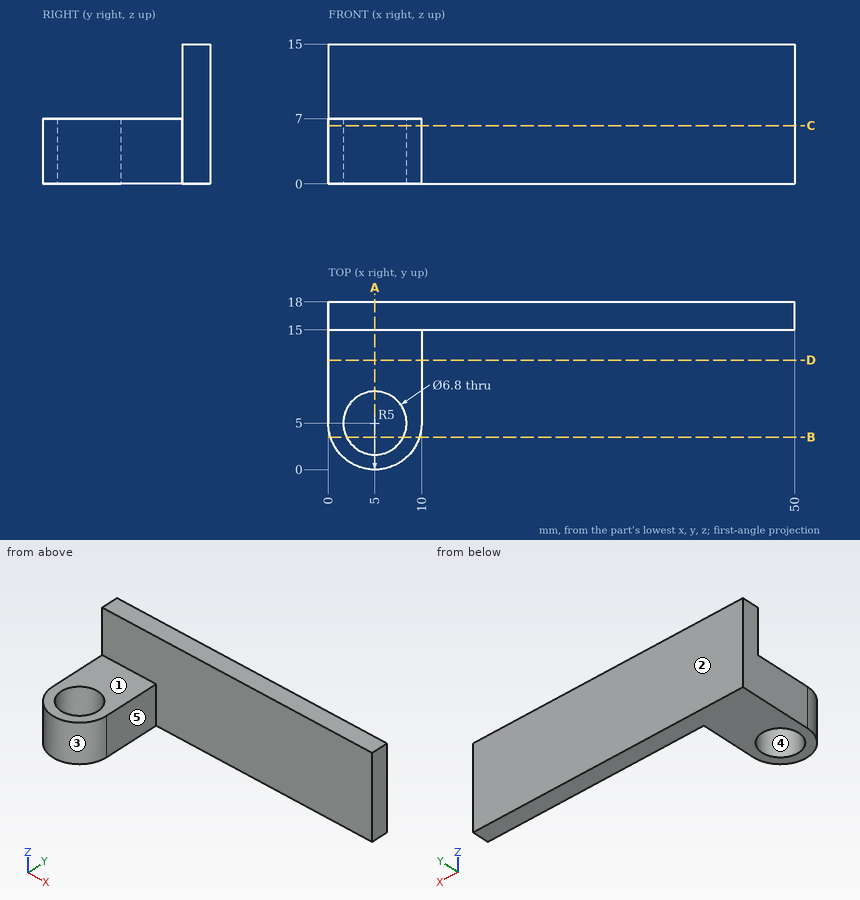
Geometry check sheet. Reference: drawing and pictorial views, mm from the part's lowest x, y, z. A direction names the side the tool comes from. Round coordinates to 2 decimals unless told otherwise and drop trailing zeros. Loops run counter-clockwise (first coordinate to the right, second up) from the corner with the lowest first, then second, coordinate; pieces in that order, holes last. Notation, with made-up numbers: (75.25, 88) - (95.25, 88) arc R15 ccw to (95.25, 107) - close; hole circle Ø3 at (87.5, 88.25). An arc over 180 degrees is marked (long way). Use a Markdown table: item, result. Add a question column.
1. Section check A-A, the plane x = 5. Record the boundary of the cut face in (y, z), plus the area to 3 significant figures.
2. Access from +Z, -Z, +X, -X, +Y, -Y to the whole of each face (thin tool, end or side, straight path). Record for the marked faces 1 and 2.
3. Section check D-D, the plane y = 11.75. Record the boundary of the cut face in (x, z).
4. Section check C-C, the plane z = 6.25. Record the boundary of the cut face in (x, y).
5. Section check B-B, the plane y = 3.5. Record the boundary of the cut face in (x, z).
6. Gauge pin test, flat ends, axial feed: pin 1 (7.5 mm diameter, centred on y = 12, z = 2.5, fed in from +X); pin 2 (6 mm diameter, centred on y = 2, z = 11.5, fed in from -X); pin 3 (1 mm diameter, centred on x = 23.5, z = 11.5, fed in from -Y); pin 4 (5 mm diameter, centred on x = 4.5, y = 6.5, fed in from +Z). Record the tip position at first contact, or that the pin passes through.
7. Release check for a two-part mould opening along X. For the marked faces 3, 4 and 5 record: released by +X, released by -X, zero draft, split by the parting line, or undercut.
8. Thickness scan on probe 1 along Y at (x, z) = (5, 5); probe 2 along X at (y, z) = (14.5, 3.75); probe 3 along Y at (x, z) = (15, 7.5). Record the ranges inside material, lowest first. Write a range as [from, to].
Checks:
| question | item | result |
|---|---|---|
| 1 | outline | (0, 0) - (1.6, 0) - (1.6, 7) - (0, 7) - close; (8.4, 0) - (18, 0) - (18, 15) - (15, 15) - (15, 7) - (8.4, 7) - close |
| 1 | area | 102 mm^2 |
| 2 | face 1 | +Z, +X, -X, -Y |
| 2 | face 2 | +Z, -Z, +X, -X, +Y |
| 3 | outline | (0, 0) - (10, 0) - (10, 7) - (0, 7) - close |
| 4 | outline | (0, 5) arc R5 ccw to (10, 5) - (10, 15) - (50, 15) - (50, 18) - (0, 18) - close; hole circle Ø6.8 at (5, 5) |
| 5 | outline | (0.23, 0) - (1.95, 0) - (1.95, 7) - (0.23, 7) - close; (8.05, 0) - (9.77, 0) - (9.77, 7) - (8.05, 7) - close |
| 6 | pin 1 | stops at x = 50 |
| 6 | pin 2 | passes through |
| 6 | pin 3 | stops at y = 15 |
| 6 | pin 4 | stops at z = 7 |
| 7 | face 3 | split by the parting line |
| 7 | face 4 | undercut |
| 7 | face 5 | released by +X |
| 8 | probe 1 | y = [0, 1.6], [8.4, 18] |
| 8 | probe 2 | x = [0, 10] |
| 8 | probe 3 | y = [15, 18] |
